```python
from build123d import *

# Parameters (mm, degrees)
EXTRUDE_2_DEPTH = 4
EXTRUDE_3_DEPTH = 3
SKETCH_5_W      = 420
SKETCH_5_H      = 10
EXTRUDE_4_DEPTH = 5
EXTRUDE_5_DEPTH = 4
EXTRUDE_6_DEPTH = 3


with BuildPart() as part:
    # 草图2 → 凸台-拉伸2 (new body)
    with BuildSketch(Plane(origin=(0, 0, 0), x_dir=(1, 0, 0), z_dir=(0, 1, 0))):
        Polygon((-130.641446974, -36.925945051), (289.358553026, -36.925945051), (284.358553026, -31.925945051), (-125.641446974, -31.925945051), align=None)
    extrude(amount=EXTRUDE_2_DEPTH)

    # 草图3 → 凸台-拉伸3 (add)
    with BuildSketch(Plane(origin=(0, 4, 0), x_dir=(1, 0, 0), z_dir=(0, 1, 0))):
        Polygon((-130.641446974, -36.925945051), (-120.641446974, -26.925945051), (279.358553026, -26.925945051), (289.358553026, -36.925945051), align=None)
    extrude_3 = extrude(amount=EXTRUDE_3_DEPTH)

    # 镜向1: 凸台-拉伸3 across plane
    add(extrude_3.mirror(Plane.ZX.offset(2)))

    # 草图5 → 凸台-拉伸4 (add)
    with BuildSketch(Plane.XY.offset(36.925945051)):
        with Locations((79.358553026, 2)):
            Rectangle(SKETCH_5_W, SKETCH_5_H)
    extrude(amount=EXTRUDE_4_DEPTH)

    # 草图7 → 凸台-拉伸5 (add)
    with BuildSketch(Plane.XY.offset(41.925945051)):
        Polygon((-130.641446974, 7), (289.358553026, 7), (284.358553026, 12), (-125.641446974, 12), align=None)
    extrude(amount=-EXTRUDE_5_DEPTH)

    # 草图8 → 凸台-拉伸6 (add)
    with BuildSketch(Plane(origin=(0, 0, 37.925945051), x_dir=(-1, 0, 0), z_dir=(0, 0, -1))):
        Polygon((-289.358553026, 7), (-279.358553026, 17), (120.641446974, 17), (130.641446974, 7), align=None)
    extrude_6 = extrude(amount=EXTRUDE_6_DEPTH)

    # 镜向2: 凸台-拉伸6 across plane
    add(extrude_6.mirror(Plane(origin=(0, 0, 39.925945051), x_dir=(1, 0, 0), z_dir=(0, 0, -1))))


solid = part.part
```
The listing builds one solid part. Answer for the finished solid, in the listing's coordinates (mm). A direction names the side the tool comes from. Coordinates: 2 decimals unless noted, no trailing zeros. Loops run counter-clockwise (first coordinate to the right, second up) from the corner with the lowest first, then second, coordinate; pieces in that order, holes last. Notation, with made-up numbers: (27.5, 81.5) -> (54.5, 81.5) arc R8 cw to (54.5, 92.5) -> close; hole circle Ø11 at (1.5, 86). An arc over 180 degrees is marked (long way). Use one line per item in the form item = value. Start each with the question number.
Item 1: A tool of negligible diameter and unlimited length cuts with its end or side. For faces 1 (the face through (-126.823, 2.07, 33.107)), 2 (the face through (76, 2, 41.926)), 3 (the face through (76, 7, 31)), from which of +Z, -Z, +X, -X, +Y, -Y can it reach the whole face along a straight path? Write none if from no direction.
Item 2: Flat-ended cylindrical pins translate along their axes: pin 1 Ø1.5 at (x, y) = (-69.5, 9.5) entering from -Z; pin 2 Ø2.5 at (x, z) = (59.5, 31.5) entering from +Y. Find the tip coordinate at first contact, or state that the pin passes through.
Item 3: Consider L1, parallel to Z at x = 265, y = 15.5; L2, parallel to Y at x = 101, z = 29.75; L3, parallel to Y at x = -14, z = 41.5. Determine where each line is inside the solid, lowest interval first. Write a range as [from, to].
Item 4: The part is cut by section A-A on x = 152.5. Determine the outline of the cut face in (y, z), then the cut area to 3 significant figures.
Answer key:
q1.face_1 = -Z, -X, -Y
q1.face_2 = +Z, +X, -X, -Y
q1.face_3 = -Z, +X, -X, +Y
q2.pin_1 = 34.93
q2.pin_2 = 7
q3.L1 = [34.93, 37.93], [41.93, 44.93]
q3.L2 = [-3, 0], [4, 7]
q3.L3 = [-3, 12]
q4.outline = (-3, 26.93) -> (0, 26.93) -> (0, 31.93) -> (4, 31.93) -> (4, 26.93) -> (7, 26.93) -> (7, 34.93) -> (17, 34.93) -> (17, 37.93) -> (12, 37.93) -> (12, 41.93) -> (17, 41.93) -> (17, 44.93) -> (7, 44.93) -> (7, 41.93) -> (-3, 41.93) -> close
q4.area = 210 mm2
